from build123d import *

# Parameters (mm, degrees)
F0_R     = 5.5
F0_R_2   = 4
F4_DEPTH = 5
F5_R     = 0.25
F6_R     = 0.25
F1_R     = 5.5
F1_R_2   = 4.25
F2_DEPTH = 2


# Not quite as in the source:
# - a fillet or chamfer that OpenCascade refuses, or shapes differently, is made with other operations: its cross-section is extruded or revolved along the edge and cut away or added


with BuildPart() as f4:
    # F0 (on Front) → F4 (new body)
    with BuildSketch(Plane.XZ):
        Circle(F0_R)
        Circle(F0_R_2, mode=Mode.SUBTRACT)
    extrude(amount=F4_DEPTH)

    # F5
    f5_edges = [f4.edges().sort_by_distance(p)[0] for p in [
        (-4, -5, 0),
    ]]
    fillet(f5_edges, radius=F5_R)

    # F6
    f6_edges = [f4.edges().sort_by_distance(p)[0] for p in [
        (-5.5, -5, 0),
    ]]
    fillet(f6_edges, radius=F6_R)

    # F1 (on face) → F2 (cut)
    with BuildSketch(Plane(origin=(0, 0, 0), x_dir=(-1, 0, 0), z_dir=(0, 1, 0))):
        Circle(F1_R)
        Circle(F1_R_2, mode=Mode.SUBTRACT)
    extrude(amount=-F2_DEPTH, mode=Mode.SUBTRACT)

    # F3: fillet of radius 2.18 on 1 edges, made by hand

    # F3_s1 → F3_t2 (revolve)
    with BuildSketch(Plane.XY):
        with BuildLine():
            ThreePointArc((-4.25, -0.0283255847), (-4.5888318925, -1.1955873377), (-5.5, -2))
            Line((-5.5, -2), (-5.4814, -2.0394334883))
            ThreePointArc((-5.4814, -2.0394334883), (-4.875, -2.0436), (-4.25, -2.0436))
            Line((-4.25, -2.0436), (-4.2064, -2))
            Line((-4.2064, -2), (-4.2064, -0.0283255847))
            Line((-4.2064, -0.0283255847), (-4.25, -0.0283255847))
        make_face()
    revolve(axis=Axis((0, -2, 0), (0, 1, 0)))


solid = f4.part
CAD build for the part. Positions are in the model's coordinates, mm. Round coordinates to 2 decimals unless told otherwise and drop trailing zeros. Write each loop counter-clockwise with the first axis right and the second up, starting at its lowest first coordinate (ties: lowest second). Pieces come first, ordered by that corner, then holes.
(1) Probe line 1 along X through (y, z) = (-0.75, -0.25); line 2 along Z through (x, y) = (0, -2.65); line 3 along Z through (x, y) = (-2.25, -0.25). List the from-to ranges inside material, lowest first.
(2) Slice it at C-C, the plane y = -0.8. Write the cut outline in (x, z).
(3) Drop flat-ended pins along their axis: P1, Ø3, axis at y = -4, z = 3.5, coming from the +X side; P2, Ø3, axis at x = 0, z = 0.5, coming from the +Y side. Give the stop position or say it passes through.
(4) Mould opens along X. For faces 1 (the face through (2, -5, -4)), 2 (the face through (-0.867, -2.342, -3.905)), 3 (the face through (-1.19, -3.36, -5.37)) say: pulls with the +X half, pulls with the -X half, needs draft (parallel to the pull), parting line crosses it, or undercut.
(5) Slice it at D-D, the plane y = -4. Write the cut outline in (x, z), and give its area (3 significant figures).
From the geometry:
1. line 1: x = -4.37 to -3.99, 3.99 to 4.37
1. line 2: z = -5.5 to -4, 4 to 5.5
1. line 3: z = -3.62 to -3.31, 3.31 to 3.62
2. outline: circle Ø8.78 at (0, 0); hole circle Ø8 at (0, 0)
3. P1: stops at x = 5.12
3. P2: passes through
4. face 1: needs draft
4. face 2: undercut
4. face 3: parting line crosses it
5. outline: circle Ø11 at (0, 0); hole circle Ø8 at (0, 0)
5. area: 44.8 mm2
